Verification items for the finished model (mm, model axes). A direction names the side the tool comes from. Give positions to 0.01 mm unless a question says otherwise; leave off trailing zeros. Write each loop counter-clockwise with the first axis right and the second up, starting at its lowest first coordinate (ties: lowest second). Pieces come first, ordered by that corner, then holes. Notation, with made-up numbers: (-23.5, 77.5) - (-6.5, 77.5) arc R9 ccw to (-6.5, 85.5) - close; hole circle Ø2 at (-14.5, 54.25). An arc over 180 degrees is marked (long way). Put each result on its own line as item: value.
from build123d import *

# Parameters (mm, degrees)
SKETCH1_W           = 38.1
SKETCH1_H           = 20.32
BOSS_EXTRUDE1_DEPTH = 2.54
SKETCH2_W           = 38.1
SKETCH2_H           = 5.08
BOSS_EXTRUDE2_DEPTH = 5.588
CHAMFER1_SIZE       = 6.35
CHAMFER1_SIZE2      = 2.311210988


with BuildPart() as part:
    # Sketch1 → Boss-Extrude1 (new body)
    with BuildSketch(Plane(origin=(0, 0, 0), x_dir=(1, 0, 0), z_dir=(0, 1, 0))):
        with Locations((2.513541667, -5.051275362)):
            Rectangle(SKETCH1_W, SKETCH1_H)
    extrude(amount=BOSS_EXTRUDE1_DEPTH)

    # Sketch2 → Boss-Extrude2 (add)
    with BuildSketch(Plane(origin=(0, 0, 0), x_dir=(1, 0, 0), z_dir=(0, 1, 0))):
        with Locations((2.513541667, 7.648724638)):
            Rectangle(SKETCH2_W, SKETCH2_H)
        with Locations((2.513541667, -17.751275362)):
            Rectangle(SKETCH2_W, SKETCH2_H)
    extrude(amount=BOSS_EXTRUDE2_DEPTH)

    # Chamfer1
    chamfer1_edges = [part.edges().sort_by_distance(p)[0] for p in [
        (2.513541667, 0, -10.188724638),
        (2.513541667, 0, 20.291275362),
    ]]
    chamfer1_side = [part.faces().sort_by_distance(p)[0] for p in [
        (2.513541667, 0, 5.051275362),
    ]]
    chamfer(chamfer1_edges, length=CHAMFER1_SIZE, length2=CHAMFER1_SIZE2, reference=chamfer1_side[0])


solid = part.part
Q1. Section check B-B, the plane x = -5.5. Record the cut outline in (y, z), plus the area to 3 significant figures.
Answers follow:
outline: (0, -3.84) - (2.31, -10.19) - (5.59, -10.19) - (5.59, -5.11) - (2.54, -5.11) - (2.54, 15.21) - (5.59, 15.21) - (5.59, 20.29) - (2.31, 20.29) - (0, 13.94) - close
area: 93.7 mm2
Q2. Section check C-C, the plane z = 3. Record the cut outline in (x, y).
Answers follow:
outline: (-16.54, 0) - (21.56, 0) - (21.56, 2.54) - (-16.54, 2.54) - close
Q3. Release check for a two-part mould opening along Z. For faces 3 (the face through (2, 4, -5.109)), 4 (the face through (2, 4, 20.291)), 5 (the face through (2, 2.54, 5)), 6 (the face through (2, 0, 5)) record: released by +Z, released by -Z, zero draft, split by the parting line, or undercut.
Answers follow:
face 3: undercut
face 4: released by +Z
face 5: undercut
face 6: zero draft
Q4. Go/stop test with a flat-tipped pin: pin 1 Ø6 at (x, z) = (7.5, 10) entering from +Y. Record where the tip stops, or that it passes through.
Answers follow:
pin 1: stops at y = 2.54
Q5. Set-up check for faces 1 (the face through (2, 5.588, -8)), 2 (the face through (2, 4, 15.211)): record each of +Z, -Z, +X, -X, +Y, -Y from which the full face is reachable in a straight line by a thin tool's end or side.
Answers follow:
face 1: +Z, -Z, +X, -X, +Y
face 2: +X, -X, +Y
Q6. Scan lines: line 1 along Z through (x, y) = (17.5, 3.7); line 2 along Y through (x, z) = (3, -3); line 3 along Y through (x, z) = (13.5, 18). Record each from-to range of solid material in increasing order.
Answers follow:
line 1: z = -10.19 to -5.11, 15.21 to 20.29
line 2: y = 0 to 2.54
line 3: y = 1.48 to 5.59
Q7. Section check D-D, the plane y = 0.95. Record the cut outline in (x, z), plus the area to 3 significant figures.
Answers follow:
outline: (-16.54, -6.45) - (21.56, -6.45) - (21.56, 16.55) - (-16.54, 16.55) - close
area: 876 mm2
Q8. Section check A-A, the plane y = 2.95. Record the cut outline in (x, z), plus the area to 3 significant figures.
Answers follow:
outline: (-16.54, -10.19) - (21.56, -10.19) - (21.56, -5.11) - (-16.54, -5.11) - close; (-16.54, 15.21) - (21.56, 15.21) - (21.56, 20.29) - (-16.54, 20.29) - close
area: 387 mm2
